from build123d import *

# Parameters (mm, degrees)
F1_DEPTH = 8.255
F2_R     = 19.05
F2_R_2   = 16.66875
F3_DEPTH = 25.4
F4_R     = 3.175
F5_DEPTH = 1.651
F6_W     = 38.1
F6_H     = 34.925
F6_R     = 11.1125
F7_DEPTH = 8.255
F8_R     = 4.7625
F9_R     = 0.79375


with BuildPart() as f1:
    # F0 (on Top) → F1 (new body)
    with BuildSketch(Plane.XY):
        with BuildLine():
            ThreePointArc((31.75, 0), (22.45064, 22.45064), (0, 31.75))
            ThreePointArc((0, 31.75), (-22.45064, 22.45064), (-31.75, 0))
            Line((-31.75, 0), (-31.75, -76.2))
            Line((-31.75, -76.2), (0, -76.2))
            Line((0, -76.2), (31.75, -76.2))
            Line((31.75, -76.2), (31.75, 0))
        make_face()
    extrude(amount=-F1_DEPTH)

    # F2 (on face) → F3 (join)
    with BuildSketch(Plane.XY):
        Circle(F2_R)
        Circle(F2_R_2, mode=Mode.SUBTRACT)
    extrude(amount=F3_DEPTH)

    # F4 (on face) → F5 (cut)
    with BuildSketch(Plane.XZ.offset(76.2)):
        with Locations((-25.4, -4.1275)):
            Circle(F4_R)
        with Locations((0, -4.1275)):
            Circle(F4_R)
        with Locations((25.4, -4.1275)):
            Circle(F4_R)
    extrude(amount=-F5_DEPTH, mode=Mode.SUBTRACT)

    # F6 (on face) → F7 (cut, through all)
    with BuildSketch(Plane.XY):
        with Locations((0, -45.72)):
            Rectangle(F6_W, F6_H)
        Circle(F6_R)
    extrude(amount=-F7_DEPTH, mode=Mode.SUBTRACT)

    # F8
    f8_edges = [f1.edges().sort_by_distance(p)[0] for p in [
        (-19.05, 0, 0),
        (-16.66875, 0, 0),
        (-19.05, -28.2575, -4.1275),
        (19.05, -28.2575, -4.1275),
        (-19.05, -63.1825, -4.1275),
        (19.05, -63.1825, -4.1275),
    ]]
    fillet(f8_edges, radius=F8_R)

    # F9
    f9_edges = [f1.edges().sort_by_distance(p)[0] for p in [
        (-19.05, 0, 25.4),
        (-16.66875, 0, 25.4),
        (-31.75, -38.1, 0),
    ]]
    fillet(f9_edges, radius=F9_R)


solid = f1.part
Here's how the part is built. I have some questions about the finished solid (model axes, mm). A direction names the side the tool comes from. Round coordinates to 2 decimals unless told otherwise and drop trailing zeros. Write each loop counter-clockwise with the first axis right and the second up, starting at its lowest first coordinate (ties: lowest second). Pieces come first, ordered by that corner, then holes. Notation, with made-up numbers: (33, -34.75) -> (48, -34.75) arc R25 ccw to (48, 3.25) -> close; hole circle Ø7 at (-39.5, 78). An arc over 180 degrees is marked (long way). One line per item, written item: value.
1) I'm going to push flat-ended pins straight in: pin 1 Ø1.9 at (x, z) = (-24, -4.5) entering from -Y; pin 2 Ø2 at (y, z) = (6, 6) entering from -X; pin 3 Ø3 at (x, y) = (2.5, -62) entering from +Z. Where does each tip first touch, or does it pass through?
Filled sheet:
pin 1: stops at y = -74.55
pin 2: stops at x = -18.38
pin 3: stops at z = 0
2) Suppose I cut it at B-B on z = 22. List the corners of the cut face in (x, y) for me.
Filled sheet:
outline: circle Ø38.1 at (0, 0); hole circle Ø33.34 at (0, 0)
3) We'd pull the mould along X, two halves only. Please class faces 4 (the face through (13, -22, 0)), 5 (the face through (15.9, 5, 14.5)), 6 (the face through (-15.12, -11.59, 14.55)), 7 (the face through (-22.372, -75.386, -3.174)): released by +X, released by -X, zero draft, split by the parting line, or undercut.
Filled sheet:
face 4: zero draft
face 5: undercut
face 6: split by the parting line
face 7: undercut
4) If I drill on line 1 (Y direction, x = 3, z = -7); line 2 (Z direction, x = -25.4, y = -75.4) (1 decimal); line 3 (X direction, y = -49, z = -5.5), over which ranges is the centre line in solid material (lowest first)? Write a range as [from, to].
Filled sheet:
line 1: y = [-76.2, -63.18], [-28.26, -10.7], [10.7, 31.61]
line 2: z = [-8.3, -7.3], [-1, 0]
line 3: x = [-31.75, -19.05], [19.05, 31.75]
5) For faces 1 (the face through (25, -74.549, -4)), 2 (the face through (31.75, -39, -4)), 3 (the face through (19.05, -46, -4)), which set-ups out of +Z, -Z, +X, -X, +Y, -Y let a thin tool reach every point of the face, with its end or its side?
Filled sheet:
face 1: -Y
face 2: +Z, -Z, +X, +Y, -Y
face 3: +Z, -Z
6) Suppose I cut it at C-C on z = 3. List the corners of the cut face in (x, y) for me.
Filled sheet:
outline: circle Ø38.78 at (0, 0); hole circle Ø32.66 at (0, 0)
